```python
from build123d import *

# Parameters (mm, degrees)
AXLE_ENVELOPE_START = -75
SKETCH_1_R          = 8.5
SKETCH_1_R_2        = 3
AXLE_ENVELOPE_DEPTH = 155
AXLE_KEYWAY_START   = -30
SKETCH_2_W          = 5
SKETCH_2_H          = 5
AXLE_KEYWAY_DEPTH   = 12.5


with BuildPart() as part:
    # Эскиз1 → Axle_envelope (new body)
    with BuildSketch(Plane.XY.offset(AXLE_ENVELOPE_START)):
        Circle(SKETCH_1_R)
        Circle(SKETCH_1_R_2, mode=Mode.SUBTRACT)
    extrude(amount=AXLE_ENVELOPE_DEPTH)

    # Эскиз2 → Axle_keyway (cut)
    with BuildSketch(Plane.XY.offset(AXLE_KEYWAY_START)):
        with Locations((8, 0)):
            Rectangle(SKETCH_2_W, SKETCH_2_H)
    extrude(amount=AXLE_KEYWAY_DEPTH, mode=Mode.SUBTRACT)


solid = part.part
```
Verification items for the finished model (mm, model axes). A direction names the side the tool comes from. Give positions to 0.01 mm unless a question says otherwise; leave off trailing zeros. Order: outer loops, then holes, each group sorted by start corner. A loop starts at its lowest first (then second) coordinate and runs counter-clockwise, first axis right, second up. Notation, with made-up numbers: M -4.75,85 L 27.25,85 A22 cw 27.25,95 Z; hole C -28.5,-8 d11. An arc over 180 degrees is marked long. Return JSON: item names as keys, results as strings. Group by question number.
1) Access from +Z, -Z, +X, -X, +Y, -Y to the whole of each face (thin tool, end or side, straight path). Record for faces 1 (the face through (7, 0, -17.5)), 2 (the face through (4, 0, 80)).
2) Go/stop test with flat-tipped pins: pin 1 Ø1.5 at (y, z) = (-0.5, -24.5) entering from +X; pin 2 Ø0.8 at (x, z) = (7, -21.5) entering from -Y; pin 3 Ø2 at (x, z) = (7.5, -24.5) entering from +Y. Record where each tip stops, or that it passes through.
3) Section check D-D on x = -5.5. Record the cut outline in (y, z).
4) Section check C-C on z = 24.5. Record the cut outline in (x, y), and give its area (3 significant figures).
5) Section check B-B on x = 0. Record the cut outline in (y, z).
6) Mould release check, pull along Z, two halves, no side actions. Record for faces 3 (the face through (7, -2.5, -24)), 4 (the face through (4, 0, -75)), 5 (the face through (-3, 0, 1)): pulls with the +Z half, pulls with the -Z half, needs draft (parallel to the pull), parting line crosses it, or undercut.
7) Section check A-A on y = 0. Record the cut outline in (x, z).
8) Scan lines: line 1 (Z direction, x = 6.75, y = -1.25); line 2 (Y direction, x = 0, z = 12); line 3 (Y direction, x = -0.75, z = 33). Record each from-to range of solid material in increasing order.
Answer block:
{
 "1": {"face 1": "+X", "face 2": "+Z, +X, -X, +Y, -Y"},
 "2": {"pin 1": "stops at x = 5.5", "pin 2": "stops at y = -5.36", "pin 3": "stops at y = 5.48"},
 "3": {"outline": "M -6.48,-75 L 6.48,-75 L 6.48,80 L -6.48,80 Z"},
 "4": {"outline": "C 0,0 d17; hole C 0,0 d6", "area": "199 mm^2"},
 "5": {"outline": "M -8.5,-75 L -3,-75 L -3,80 L -8.5,80 Z; M 3,-75 L 8.5,-75 L 8.5,80 L 3,80 Z"},
 "6": {"face 3": "undercut", "face 4": "pulls with the -Z half", "face 5": "needs draft"},
 "7": {"outline": "M -8.5,-75 L -3,-75 L -3,80 L -8.5,80 Z; M 3,-75 L 8.5,-75 L 8.5,-30 L 5.5,-30 L 5.5,-17.5 L 8.5,-17.5 L 8.5,80 L 3,80 Z"},
 "8": {"line 1": "z = -75 to -30, -17.5 to 80", "line 2": "y = -8.5 to -3, 3 to 8.5", "line 3": "y = -8.47 to -2.9, 2.9 to 8.47"}
}
